Autodesk Inventor part; units mm, degrees
ref_plane "YZ Plane" through (0, 0, 0) normal (1, 0, 0) x (0, 1, 0)
ref_plane "XZ Plane" through (0, 0, 0) normal (0, 1, 0) x (-1, 0, 0)
ref_plane "XY Plane" through (0, 0, 0) normal (0, 0, 1) x (1, 0, 0)
sketch "Sketch2" plane through (0, 0, 0) normal (0, 0, 1) x (1, 0, 0)
  line L0 (1, 2.5) -> (1, 5.5)
  line L1 (1, 5.5) -> (3, 5.5)
  line L2 (3, 5.5) -> (3, 7.5)
  line L3 (3, 7.5) -> (5.75, 7.5)
  line L4 (5.75, 7.5) -> (10, 2.5)
  line L5 (10, 2.5) -> (10, 0)
  line L6 (1, 2.5) -> (5.75, 2.5)
  line L7 (5.75, 2.5) -> (5.75, 0)
  line L8 (5.75, 0) -> (10, 0)
  line L9 (0, 0) -> (0, 19.425)
  dimension "d0" = 6
  dimension "d1" = 2
  dimension "d2" = 11.5
  dimension "d3" = 20
  dimension "d4" = 2.5
  dimension "d5" = 3
  dimension "d6" = 2
revolve "Revolution1" add sketch "Sketch2" angle 360 about axis through (0, 0, 0) along (0, 1, 0)
sketch "Sketch3" plane through (0, 7.5, 0) normal (0, 1, 0) x (1, 0, 0)
  point P0 (0, 0)
  point P1 (0, 7.5)
  dimension "d8" = 7.5
hole "Hole1" at (0, 7.5, -7.5) direction (0, -1, 0) diameter 2.9 end through all counterbore diameter 5.5 counterbore depth 3.5
pattern_circular "Circular Pattern1" count 3 over 360 about axis through (0, -10, 0) along (0, 1, 0) of "Hole1"
properties part number "902-4250 magnet hold"
Model file for the job. Use its own axes, mm. A direction names the side the tool comes from. Coordinates: 2 decimals unless noted, no trailing zeros. Write each loop counter-clockwise with the first axis right and the second up, starting at its lowest first coordinate (ties: lowest second). Pieces come first, ordered by that corner, then holes. Notation, with made-up numbers: (9, 47) - (46, 47) arc R20 ccw to (46, 58) - close; hole circle Ø7 at (53.25, 55). An arc over 180 degrees is marked (long way). Write each question's results on one line, items separated by ' | '. Start each with the question number.
1) Probe line 1 along Z through (x, y) = (0, 1.5); line 2 along Z through (x, y) = (0, 2.75); line 3 along X through (y, z) = (2.8, 3.75). List the from-to ranges inside material, lowest first. Write a range as from..to.
2) Flat gauge pins, fed straight in: P1, Ø2.5, axis at x = 0, z = 0, coming from the +Y side; P2, Ø5, axis at x = 0, z = -7.5, coming from the +Y side; P3, Ø2, axis at x = -7, y = 6, coming from the +Z side; P4, Ø2.5, axis at x = 0, z = -7.5, coming from the -Y side. Where does each tip first touch, or does it go through?
3) Cut at C-C (y = 2). Write the cut outline in (x, z) (3 decimals), then the cut area to 3 significant figures.
4) Cut at A-A (z = 0). Write the cut outline in (x, y), then the cut area to 3 significant figures.
5) Mould opens along X. For faces 1 (the face through (-2.17, 1.23, -9.76)), 2 (the face through (-3, 7.5, -2)), 3 (the face through (5, 4, 3)) say: pulls with the +X half, pulls with the -X half, needs draft (parallel to the pull), parting line crosses it, or undercut.
6) 3-axis set-ups, long thin cutter, end or side, ignore diameter. For faces 4 (the face through (-0.44, 1.97, -6.12)), 5 (the face through (-5, 4, 3)), 6 (the face through (-0.75, 1.23, 5.7)): which of +Z, -Z, +X, -X, +Y, -Y reach the whole face in a straight line?
Returned:
1) line 1: -10..-8.95, -6.05..-5.75, 5.75..10 | line 2: -9.79..-8.95, -6.05..-1, 1..9.79 | line 3: -8.99..-7.95, -5.05..5.05, 7.95..8.99
2) P1: y = 5.5 | P2: y = 4 | P3: z = 1.23 | P4: through
3) outline: circle Ø20 at (0, 0); hole circle Ø2.9 at (-6.495, 3.75); hole circle Ø11.5 at (0, 0); hole circle Ø2.9 at (0, -7.5); hole circle Ø2.9 at (6.495, 3.75) | area: 190 mm^2
4) outline: (-10, 0) - (-5.75, 0) - (-5.75, 2.5) - (-1, 2.5) - (-1, 5.5) - (-3, 5.5) - (-3, 7.5) - (-5.75, 7.5) - (-10, 2.5) - close; (1, 2.5) - (5.75, 2.5) - (5.75, 0) - (10, 0) - (10, 2.5) - (5.75, 7.5) - (3, 7.5) - (3, 5.5) - (1, 5.5) - close | area: 82.0 mm^2
5) face 1: parting line crosses it | face 2: needs draft | face 3: undercut
6) face 4: +Y, -Y | face 5: +Y | face 6: -Y
